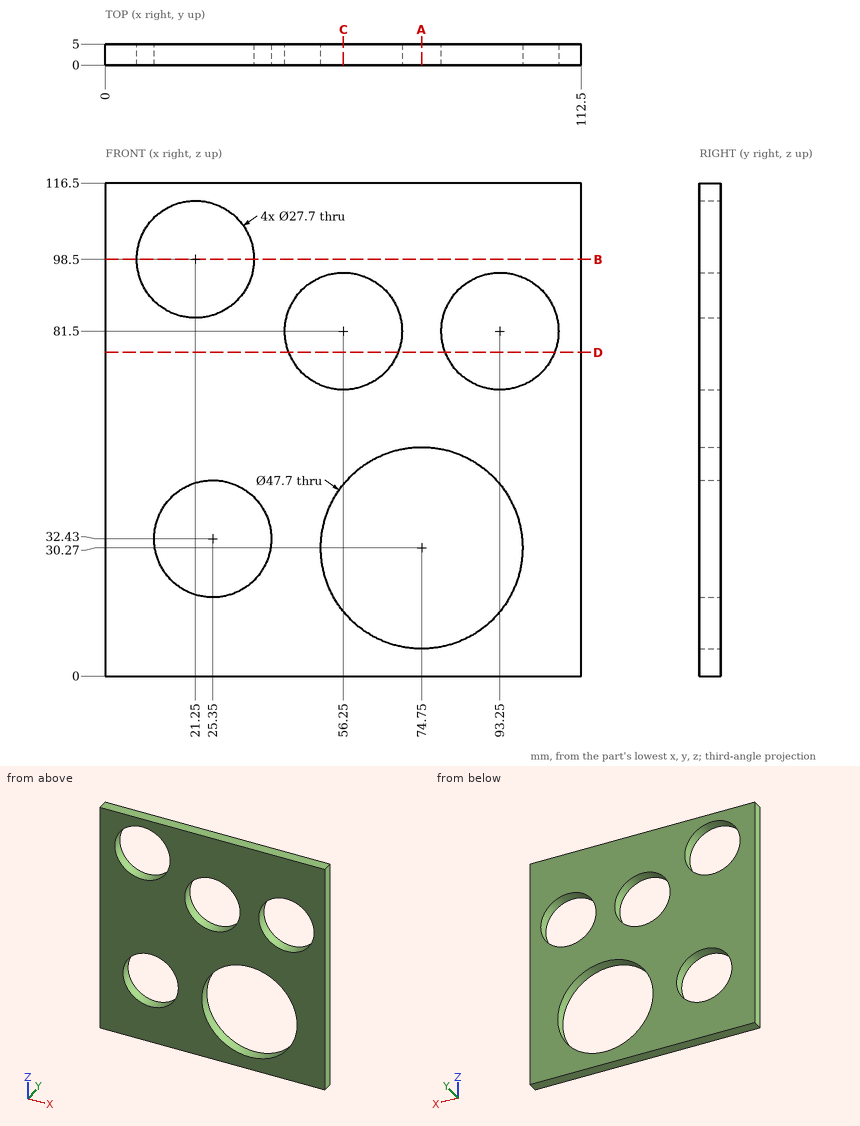
Print and shaded views of the part. All mm, measured from the part's lowest x, y and z. Give positions to 0.01 mm unless a question says otherwise; leave off trailing zeros. Loops run counter-clockwise (first coordinate to the right, second up) from the corner with the lowest first, then second, coordinate; pieces in that order, holes last.
1) Saw through at A-A (x = 74.75). Write the cut outline in (y, z).
2) Saw through at B-B (z = 98.5). Write the cut outline in (x, y), plus the area to 3 significant figures.
3) Wall check: line 1 (X direction, y = 2.55, z = 81.5); line 2 (X direction, y = 3.8, z = 90.5) (1 decimal); line 3 (X direction, y = 4, z = 34). Give the ranges that are in metal, low to high.
4) Saw through at C-C (x = 56.25). Write the cut outline in (y, z).
5) Flat gauge pin, fed straight in: pin 1 Ø16.5 at (x, z) = (56.25, 81.5) entering from +Y. Where does the tip first touch, or does it go through?
6) Saw through at D-D (z = 76.5). Write the cut outline in (x, y), plus the area to 3 significant figures.
Answer block:
1. outline: (0, 0) - (5, 0) - (5, 6.42) - (0, 6.42) - close; (0, 54.12) - (5, 54.12) - (5, 116.5) - (0, 116.5) - close
2. outline: (0, 0) - (7.4, 0) - (7.4, 5) - (0, 5) - close; (35.1, 0) - (112.5, 0) - (112.5, 5) - (35.1, 5) - close
2. area: 424 mm2
3. line 1: x = 0 to 42.4, 70.1 to 79.4, 107.1 to 112.5
3. line 2: x = 0 to 9.9, 32.6 to 45.7, 66.8 to 82.7, 103.8 to 112.5
3. line 3: x = 0 to 11.59, 39.11 to 51.19, 98.31 to 112.5
4. outline: (0, 0) - (5, 0) - (5, 15.22) - (0, 15.22) - close; (0, 45.32) - (5, 45.32) - (5, 67.65) - (0, 67.65) - close; (0, 95.35) - (5, 95.35) - (5, 116.5) - (0, 116.5) - close
5. pin 1: passes through
6. outline: (0, 0) - (43.33, 0) - (43.33, 5) - (0, 5) - close; (69.17, 0) - (80.33, 0) - (80.33, 5) - (69.17, 5) - close; (106.17, 0) - (112.5, 0) - (112.5, 5) - (106.17, 5) - close
6. area: 304 mm2
